Autodesk Inventor part; units mm, degrees
ref_plane "Plano de trabajo1" through (0, 20, 0) normal (0, 1, 0) x (-1, 0, 0)
ref_plane "YZ Plane" through (0, 0, 0) normal (1, 0, 0) x (0, 1, 0)
ref_plane "XY Plane" through (0, 0, 0) normal (0, 0, 1) x (1, 0, 0)
sketch "Boceto1" plane through (0, 0, 0) normal (0, 1, 0) x (-1, 0, 0)
  line L0 (0, 0) -> (0, -154)
  line L1 (35, -185) -> (95, -185)
  line L2 (130, -154) -> (130, 0)
  line L3 (130, 0) -> (0, 0)
  line L4 (0, 0) -> (0, -154) construction
  line L5 (65, -185) -> (95, -185) construction
  line L6 (95, -185) -> (95, -206.4869) construction
  line L7 (95, -206.4869) -> (35, -206.4869) construction
  line L8 (35, -206.4869) -> (35, -185) construction
  line L9 (0, -154) -> (35, -185)
  line L10 (95, -185) -> (130, -154)
  line L11 (61.4516, 0) -> (61.4516, -5) construction
  line L12 (130, -81.3037) -> (125, -81.3037) construction
  line L13 (0, -85.0807) -> (5, -85.0807) construction
  line L14 (125, -5) -> (5, -5)
  line L15 (5, -5) -> (5, -148.3548)
  line L16 (125, -148.3548) -> (125, -5)
  line L17 (112.5, -169.5) -> (109.1848, -165.7571) construction
  line L18 (65, -185) -> (65, -180) construction
  line L19 (17.5, -169.5) -> (20.8152, -165.7571) construction
  line L20 (20.8152, -165.7571) -> (5, -151.7493)
  line L21 (20.8152, -165.7571) -> (36.8959, -180)
  line L22 (36.8959, -180) -> (93.1041, -180)
  line L23 (93.1041, -180) -> (125, -151.7493)
  line L24 (125, -151.7493) -> (125, -148.3548)
  line L25 (5, -148.3548) -> (5, -151.7493)
  dimension "d2" = 154
  dimension "d3" = 30
  dimension "d4" = 60
  dimension "d5" = 5
  dimension "d6" = 5
  dimension "d7" = 5
  dimension "d8" = 5
  dimension "d9" = 5
  dimension "d10" = 5
extrude "Extrusión1" add sketch "Boceto1" along normal blind 3 contours L16 L24 L23 L22 L21 L20 L25 L15 L14
extrude "Extrusión2" add sketch "Boceto1" along normal blind 20
ref_plane "Plano de trabajo1" through (0, 20, 0) normal (0, 1, 0) x (-1, 0, 0)
sketch "Boceto2" plane through (0, 20, 0) normal (0, 1, 0) x (-1, 0, 0)
  line L0 (0, 0) -> (0, -154) construction
  line L1 (0, 0) -> (0, -26.749) construction
  line L2 (130, -154) -> (130, 0) construction
  line L3 (125, -151.7493) -> (93.1041, -180) construction
  line L4 (125, -151.7493) -> (5, -151.7493) construction
  line L5 (65, -151.7493) -> (65, -26.749) construction
  line L6 (125, -89.2492) -> (5, -89.2492) construction
  line L7 (5, -151.7493) -> (5, -5) construction
  line L8 (125, -26.749) -> (125, -31.749) construction
  line L9 (125, -31.749) -> (120, -31.749) construction
  line L10 (120, -31.749) -> (120, -26.749) construction
  line L11 (125, -31.749) -> (120, -26.749) construction
  line L12 (120, -31.749) -> (125, -26.749) construction
  circle A0 centre (122.5, -29.249) radius 2
  line L13 (125, -31.749) -> (125, -26.749)
  arc A1 (120, -26.749) -> (125, -31.749) centre (122.5, -29.249) ccw
  line L14 (5, -26.749) -> (5, -31.749) construction
  circle A2 centre (7.5, -29.249) radius 2
  line L15 (5, -31.749) -> (5, -26.749)
  arc A3 (5, -31.749) -> (10, -26.749) centre (7.5, -29.249) ccw
  arc A4 (125, -26.749) -> (120.5, -32.1645) centre (122.5, -29.249) ccw
  arc A5 (10.6306, -27.606) -> (5, -26.749) centre (7.5, -29.249) ccw
  line L16 (5, -26.749) -> (5, -173.4983) construction
  line L17 (125, -151.7493) -> (125, -146.7493) construction
  line L18 (120, -146.7493) -> (125, -151.7493) construction
  circle A6 centre (122.5, -149.2493) radius 2
  line L19 (125, -146.7493) -> (125, -151.7493)
  arc A7 (125, -146.7493) -> (120, -151.7493) centre (122.5, -149.2493) ccw
  arc A8 (10, -151.7493) -> (5, -146.7493) centre (7.5, -149.2493) ccw
  line L20 (5, -151.7493) -> (5, -146.7493) construction
  line L21 (5, -146.7493) -> (5, -151.7493)
  circle A9 centre (7.5, -149.2493) radius 2
  arc A10 (120.5, -146.3339) -> (125, -151.7493) centre (122.5, -149.2493) ccw
  arc A11 (5, -151.7493) -> (10.6306, -150.8923) centre (7.5, -149.2493) ccw
  point P0 (10, -151.7493)
  point P1 (10, -26.749)
  point P2 (120, -26.749)
  dimension "d16" = 26.749
  dimension "d19" = 4
extrude "Extrusión3" add sketch "Boceto2" against normal blind 17
extrude "Extrusión4" cut sketch "Boceto2" against normal through all contours A0 | A2 | A6 | A9
sketch "Boceto3" plane through (0, 3, 0) normal (0, 1, 0) x (1, 0, 0)
  line L0 (-125, 5) -> (-5, 5) construction
  line L1 (-65, 5) -> (-110, 5) construction
  line L2 (-110, 5) -> (-110, 15) construction
  line L3 (-110, 15) -> (-20, 15)
  line L4 (-20, 15) -> (-20, 145.2684)
  line L5 (-30, 155.2684) -> (-100, 155.2684)
  line L6 (-110, 145.2684) -> (-110, 15)
  line L7 (-65, 15) -> (-65, 155.2684) construction
  line L8 (-100, 155.2684) -> (-110, 145.2684)
  line L9 (-30, 155.2684) -> (-20, 145.2684)
  line L10 (-106.9205, 15) -> (-104.9205, 15)
  line L11 (-104.9205, 15) -> (-104.9205, 155.2684)
  line L12 (-106.9205, 155.2684) -> (-106.9205, 15)
  line L13 (-99.0505, 15) -> (-99.0505, 155.2684)
  line L14 (-101.0505, 155.2684) -> (-101.0505, 15)
  line L15 (-93.1805, 15) -> (-93.1805, 155.2684)
  line L16 (-95.1805, 155.2684) -> (-95.1805, 15)
  line L17 (-87.3105, 15) -> (-87.3105, 155.2684)
  line L18 (-89.3105, 155.2684) -> (-89.3105, 15)
  line L19 (-81.4405, 15) -> (-81.4405, 155.2684)
  line L20 (-83.4405, 155.2684) -> (-83.4405, 15)
  line L21 (-75.5705, 15) -> (-75.5705, 155.2684)
  line L22 (-77.5705, 155.2684) -> (-77.5705, 15)
  line L23 (-69.7005, 15) -> (-69.7005, 155.2684)
  line L24 (-71.7005, 155.2684) -> (-71.7005, 15)
  line L25 (-63.8305, 15) -> (-63.8305, 155.2684)
  line L26 (-65.8305, 155.2684) -> (-65.8305, 15)
  line L27 (-57.9605, 15) -> (-57.9605, 155.2684)
  line L28 (-59.9605, 155.2684) -> (-59.9605, 15)
  line L29 (-52.0905, 15) -> (-52.0905, 155.2684)
  line L30 (-54.0905, 155.2684) -> (-54.0905, 15)
  line L31 (-46.2205, 15) -> (-46.2205, 155.2684)
  line L32 (-48.2205, 155.2684) -> (-48.2205, 15)
  line L33 (-40.3505, 15) -> (-40.3505, 155.2684)
  line L34 (-42.3505, 155.2684) -> (-42.3505, 15)
  line L35 (-34.4805, 15) -> (-34.4805, 155.2684)
  line L36 (-36.4805, 155.2684) -> (-36.4805, 15)
  line L37 (-28.6105, 15) -> (-28.6105, 155.2684)
  line L38 (-30.6105, 155.2684) -> (-30.6105, 15)
  line L39 (-22.7405, 15) -> (-22.7405, 155.2684)
  line L40 (-24.7405, 155.2684) -> (-24.7405, 15)
  line L41 (-106.9205, 148.348) -> (-104.9205, 150.348)
  line L42 (-101.0505, 154.218) -> (-100, 155.2684)
  line L43 (-110, 145.2684) -> (-100, 155.2684)
  line L44 (-100, 155.2684) -> (-30, 155.2684)
  line L45 (-30, 155.2684) -> (-20, 145.2684)
  line L46 (-20, 145.2684) -> (-20, 15)
  line L47 (-110, 15) -> (-20, 15)
  line L48 (-110, 15) -> (-110, 145.2684)
  line L49 (-83.4405, 15) -> (-81.4405, 15)
  line L50 (-77.5705, 15) -> (-75.5705, 15)
  line L51 (-87.3105, 15) -> (-89.3105, 15)
  line L52 (-93.1805, 15) -> (-95.1805, 15)
  line L53 (-99.0505, 15) -> (-101.0505, 15)
  line L54 (-104.9205, 15) -> (-106.9205, 15)
  line L55 (-71.7005, 15) -> (-69.7005, 15)
  line L56 (-65.8305, 15) -> (-63.8305, 15)
  line L57 (-59.9605, 15) -> (-57.9605, 15)
  line L58 (-54.0905, 15) -> (-52.0905, 15)
  line L59 (-48.2205, 15) -> (-46.2205, 15)
  line L60 (-42.3505, 15) -> (-40.3505, 15)
  line L61 (-36.4805, 15) -> (-34.4805, 15)
  line L62 (-30.6105, 15) -> (-28.6105, 15)
  line L63 (-24.7405, 15) -> (-22.7405, 15)
  line L64 (-22.7405, 148.0089) -> (-24.7405, 150.0089)
  line L65 (-28.6105, 153.8789) -> (-30, 155.2684)
  line L66 (-30.6105, 155.2684) -> (-30, 155.2684)
  line L67 (-35, 185) -> (-95, 185)
  line L68 (-34.4805, 155.2684) -> (-36.4805, 155.2684)
  line L69 (-40.3505, 155.2684) -> (-42.3505, 155.2684)
  line L70 (-46.2205, 155.2684) -> (-48.2205, 155.2684)
  line L71 (-52.0905, 155.2684) -> (-54.0905, 155.2684)
  line L72 (-57.9605, 155.2684) -> (-59.9605, 155.2684)
  line L73 (-63.8305, 155.2684) -> (-65.8305, 155.2684)
  line L74 (-69.7005, 155.2684) -> (-71.7005, 155.2684)
  line L75 (-75.5705, 155.2684) -> (-77.5705, 155.2684)
  line L76 (-81.4405, 155.2684) -> (-83.4405, 155.2684)
  line L77 (-87.3105, 155.2684) -> (-89.3105, 155.2684)
  line L78 (-93.1805, 155.2684) -> (-95.1805, 155.2684)
  line L79 (-99.0505, 155.2684) -> (-100, 155.2684)
  line L80 (-101.0505, 154.218) -> (-100, 155.2684)
  line L81 (-104.9205, 150.348) -> (-106.9205, 148.348)
  line L82 (-106.9205, 148.348) -> (-104.9205, 150.348)
  point P0 (0, 0)
  dimension "d24" = 45
  dimension "d25" = 10
  dimension "d32" = 5.87
extrude "Extrusión5" cut sketch "Boceto3" against normal blind 10 contours L6 L8 L12 L3 | L11 L8 L14 L3 | L13 L5 L16 L3 | L15 L5 L18 L3 | L17 L5 L20 L3 | L19 L5 L22 L3 | L21 L5 L24 L3 | L23 L5 L26 L3 | L25 L5 L28 L3 | L27 L5 L30 L3 | L29 L5 L32 L3 | L31 L5 L34 L3 | L33 L5 L36 L3 | L35 L5 L38 L3 | L37 L9 L40 L3 | L39 L9 L4 L3
fillet "Empalme1" radius 5 4 edges at (-130, 10, 0) (0, 10, 0) (0, 10, -154) (-130, 10, -154)
fillet "Empalme2" radius 5 2 edges at (-95, 10, -185) (-35, 10, -185)
Source: CAD feature listing. Evaluate the final solid. Frame: model axes, mm. A direction names the side the tool comes from. Give positions to 0.01 mm unless a question says otherwise; leave off trailing zeros. Write each loop counter-clockwise with the first axis right and the second up, starting at its lowest first coordinate (ties: lowest second). Pieces come first, ordered by that corner, then holes. Notation, with made-up numbers: (83.5, 9) -> (133.5, 9) arc R25 ccw to (133.5, 29) -> close; hole circle Ø3 at (-5.5, 60.25). An arc over 180 degrees is marked (long way). Return JSON: item names as keys, results as strings. Group by question number.
1. Section D-D, the plane z = -174. Output: boundary loops of the cut face in (x, y), then the cut area to 3 significant figures.
2. Access query for faces 1 (the face through (-5, 11, -88)), 2 (the face through (0, 10, -77)). Directions: +Z, -Z, +X, -X, +Y, -Y. A direction counts if a zero-diameter tool reaches every point of the face in a straight line with its end or side. Return the directions, or none.
3. Section B-B, the plane y = 17. Count the separate pieces of the cut face and the enclosed holes in it, then the cut area to 3 significant figures.
4. Section A-A, the plane x = -7.5. Output: boundary loops of the cut face in (y, z), then the cut area to 3 significant figures.
5. Material intervals for line 1 (X direction, y = 18, z = -16.5); line 2 (Z direction, x = -122.5, y = 10); line 3 (Z direction, x = -63, y = 4), sorted ascending. Write a range as from..to.
6. Pin query (flat end, axial travel): pin 1 Ø1.5 at (x, z) = (-38, -67) entering from -Y; pin 2 Ø1 at (x, y) = (-111.5, 17) entering from -Z; pin 3 Ø5 at (x, z) = (-83.5, -28.5) entering from +Y. Return the tip coordinate at first contact, or that it passes through.
Determined:
{
 "1": {"outline": "(-107.42, 0) -> (-22.58, 0) -> (-22.58, 20) -> (-30.12, 20) -> (-30.12, 3) -> (-99.88, 3) -> (-99.88, 20) -> (-107.42, 20) -> close", "area": "511 mm2"},
 "2": {"face 1": "+Y", "face 2": "+Z, -Z, +X, +Y, -Y"},
 "3": {"separate pieces": "1", "enclosed holes": "5", "area": "2,950 mm2"},
 "4": {"outline": "(0, -160.64) -> (20, -160.64) -> (20, -153.96) -> (3, -153.96) -> (3, -152.78) -> (20, -152.78) -> (20, -151.25) -> (0, -151.25) -> close; (0, -147.25) -> (20, -147.25) -> (20, -145.71) -> (3, -145.71) -> (3, -32.78) -> (20, -32.78) -> (20, -31.25) -> (0, -31.25) -> close; (0, -27.25) -> (20, -27.25) -> (20, -25.71) -> (3, -25.71) -> (3, -5) -> (20, -5) -> (20, 0) -> (0, 0) -> close", "area": "761 mm2"},
 "5": {"line 1": "x = -130..-125, -5..0", "line 2": "z = -160.64..-153.96, -152.78..-151.25, -147.25..-145.71, -32.78..-31.25, -27.25..-25.71, -5..0", "line 3": "z = -185..-180, -5..0"},
 "6": {"pin 1": "passes through", "pin 2": "stops at z = -170.83", "pin 3": "stops at y = 3"}
}
